Drawing for the job (mm, zero at the part's lowest x, y, z). Round coordinates to 2 decimals unless told otherwise and drop trailing zeros. Write each loop counter-clockwise with the first axis right and the second up, starting at its lowest first coordinate (ties: lowest second). Pieces come first, ordered by that corner, then holes.
Item 1: Wall check: probe 1 along X at (y, z) = (10.75, 4.75); probe 2 along X at (y, z) = (10.5, 10.75); probe 3 along Y at (x, z) = (25, 5.5). Give the ranges that are in metal, low to high.
Item 2: Band-saw the part on D-D, the plane y = 1.75. Write the cut outline in (x, z).
Item 3: Mould opens along Y. For the marked faces 1, 2 and 3 say: +Y half, -Y half, draft (parallel to the pull), parting line (faces both ways), or undercut.
Item 4: Band-saw the part on A-A, the plane y = 10. Write the cut outline in (x, z), then the cut area to 3 significant figures.
Item 5: Band-saw the part on C-C, the plane z = 4.5. Write the cut outline in (x, y), then the cut area to 3 significant figures.
Item 6: Drop a flat-ended pin along its axis: pin 1 Ø4 at (x, y) = (25, 10) entering from -Z. Give the stop position or say it passes through.
Item 7: Band-saw the part on B-B, the plane x = 25. Write the cut outline in (y, z), then the cut area to 3 significant figures.
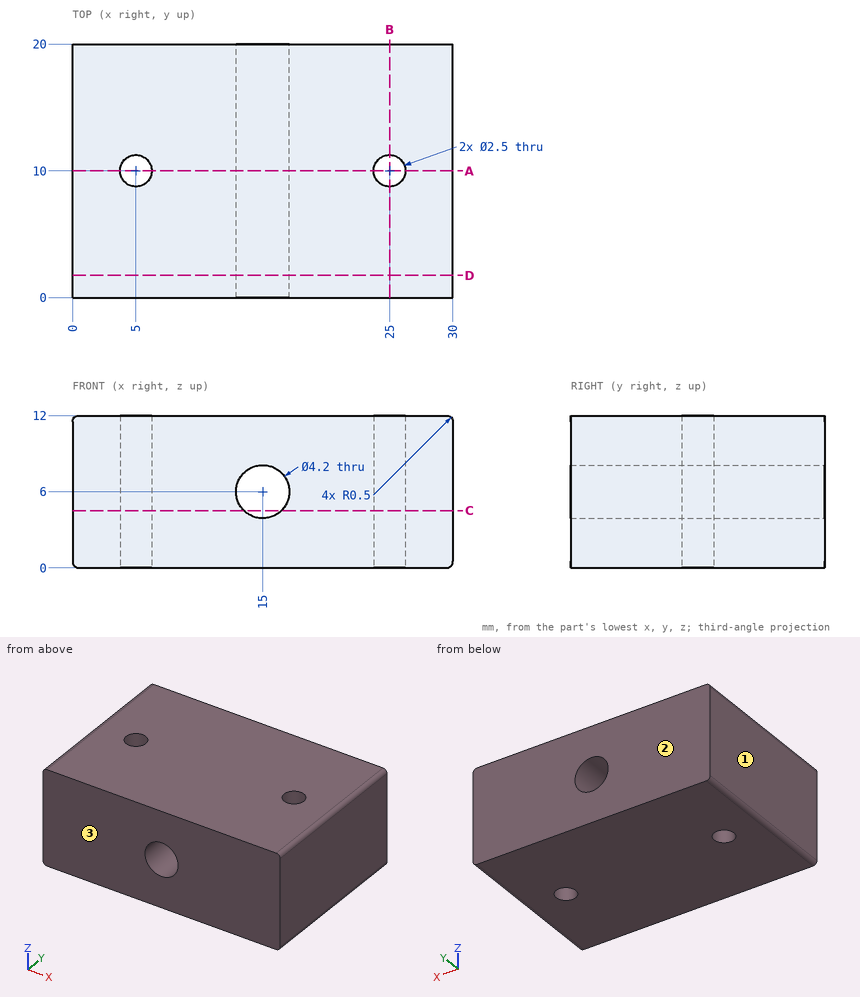
Results:
1. probe 1: x = 0 to 4, 6 to 13.31, 16.69 to 24, 26 to 30
1. probe 2: x = 0 to 3.85, 6.15 to 23.85, 26.15 to 30
1. probe 3: y = 0 to 8.75, 11.25 to 20
2. outline: (0, 0.5) arc R0.5 ccw to (0.5, 0) - (29.5, 0) arc R0.5 ccw to (30, 0.5) - (30, 11.5) arc R0.5 ccw to (29.5, 12) - (0.5, 12) arc R0.5 ccw to (0, 11.5) - close; hole circle Ø4.2 at (15, 6)
3. face 1: draft
3. face 2: +Y half
3. face 3: -Y half
4. outline: (0, 0.5) arc R0.5 ccw to (0.5, 0) - (3.75, 0) - (3.75, 12) - (0.5, 12) arc R0.5 ccw to (0, 11.5) - close; (6.25, 0) - (23.75, 0) - (23.75, 12) - (6.25, 12) - close; (26.25, 0) - (29.5, 0) arc R0.5 ccw to (30, 0.5) - (30, 11.5) arc R0.5 ccw to (29.5, 12) - (26.25, 12) - close; hole circle Ø4.2 at (15, 6)
4. area: 286 mm2
5. outline: (0, 0) - (13.53, 0) - (13.53, 20) - (0, 20) - close; (16.47, 0) - (30, 0) - (30, 20) - (16.47, 20) - close; hole circle Ø2.5 at (5, 10); hole circle Ø2.5 at (25, 10)
5. area: 531 mm2
6. pin 1: stops at z = 0
7. outline: (0, 0) - (8.75, 0) - (8.75, 12) - (0, 12) - close; (11.25, 0) - (20, 0) - (20, 12) - (11.25, 12) - close
7. area: 210 mm2
